from build123d import *

# Parameters (mm, degrees)
SKETCH1_R                 = 1.651
BOSS_EXTRUDE2_DEPTH       = 3.048
SKETCH2_R                 = 1.143
CUT_EXTRUDE1_DEPTH        = 4.048
SKETCH3_R                 = 12.1285
CUT_EXTRUDE2_DEPTH        = 4.048
SKETCH4_W                 = 28.562713242
SKETCH4_H                 = 11.677503754
BOSS_EXTRUDE3_DEPTH       = 3.048
SKETCH5_W                 = 216.7214489
SKETCH5_H                 = 130.569220634
CUT_EXTRUDE4_DEPTH        = 4.048
SKETCH6_W                 = 4.7625
SKETCH6_H                 = 27.432
CUT_EXTRUDE5_DEPTH        = 4.048
SKETCH10_W                = 11.43
SKETCH10_H                = 10.16
CUT_EXTRUDE9_DEPTH        = 4.048
FILLET1_R                 = 6
FILLET2_R                 = 6
SKETCH66_R                = 1.651
CUT_EXTRUDE65_DEPTH       = 97.79
SKETCH120_R               = 3.175
CUT_EXTRUDE119_DEPTH      = 103.378
CUT_EXTRUDE119_DEPTH_BACK = 48.768
CUT_EXTRUDE12_DEPTH       = 10
FILLET3_R                 = 2.54
BOSS_EXTRUDE4_DEPTH       = 3.048
SKETCH122_R               = 2.032
CUT_EXTRUDE120_DEPTH      = 27.305
SKETCH123_R               = 12.192
CUT_EXTRUDE121_DEPTH      = 19.05


with BuildPart() as part:
    # Sketch1 → Boss-Extrude2 (new body)
    with BuildSketch(Plane.XY):
        with BuildLine():
            Line((-64.964441474, 37.338), (-54.550441474, 37.338))
            Line((-54.550441474, 37.338), (-54.550441474, -37.338))
            Line((-54.550441474, -37.338), (-64.964441474, -37.338))
            ThreePointArc((-64.964441474, -37.338), (0, -74.93), (64.964441474, -37.338))
            Line((64.964441474, -37.338), (54.550441474, -37.338))
            Line((54.550441474, -37.338), (54.550441474, 37.338))
            Line((54.550441474, 37.338), (64.964441474, 37.338))
            ThreePointArc((64.964441474, 37.338), (0, 74.93), (-64.964441474, 37.338))
        make_face()
        with Locations((-46.482, 11.049)):
            Circle(SKETCH1_R, mode=Mode.SUBTRACT)
        with Locations((-21.083270032, 10.795)):
            Circle(SKETCH1_R, mode=Mode.SUBTRACT)
        with Locations((-21.083270032, -10.795)):
            Circle(SKETCH1_R, mode=Mode.SUBTRACT)
        with Locations((-46.482, -11.049)):
            Circle(SKETCH1_R, mode=Mode.SUBTRACT)
        with Locations((46.482, -11.049)):
            Circle(SKETCH1_R, mode=Mode.SUBTRACT)
        with Locations((21.083270032, -10.795)):
            Circle(SKETCH1_R, mode=Mode.SUBTRACT)
        with Locations((21.083270032, 10.795)):
            Circle(SKETCH1_R, mode=Mode.SUBTRACT)
        with Locations((46.482, 11.049)):
            Circle(SKETCH1_R, mode=Mode.SUBTRACT)
    extrude(amount=BOSS_EXTRUDE2_DEPTH)

    # Sketch2 → Cut-Extrude1 (cut, through all)
    with BuildSketch(Plane.XY.offset(3.048)):
        with Locations((-6.731, 62.23)):
            Circle(SKETCH2_R)
        with Locations((6.731, 62.23)):
            Circle(SKETCH2_R)
    extrude(amount=-CUT_EXTRUDE1_DEPTH, mode=Mode.SUBTRACT)

    # Sketch3 → Cut-Extrude2 (cut, through all)
    with BuildSketch(Plane(origin=(0, 0, 0), x_dir=(-1, 0, 0), z_dir=(0, 0, -1))):
        with Locations((-15.777608989, -58.882838371)):
            Circle(SKETCH3_R)
        with Locations((15.777608989, -58.882838371)):
            Circle(SKETCH3_R)
        with Locations((-43.105229381, -43.105229381)):
            Circle(SKETCH3_R)
        with Locations((19.05, 32.995567884)):
            Circle(SKETCH3_R)
        with Locations((-43.105229381, 43.105229381)):
            Circle(SKETCH3_R)
        with Locations((43.105229381, 43.105229381)):
            Circle(SKETCH3_R)
        with Locations((-19.05, 32.995567884)):
            Circle(SKETCH3_R)
        with Locations((43.105229381, -43.105229381)):
            Circle(SKETCH3_R)
    extrude(amount=-CUT_EXTRUDE2_DEPTH, mode=Mode.SUBTRACT)

    # Sketch4 → Boss-Extrude3 (add)
    with BuildSketch(Plane(origin=(0, 0, 0), x_dir=(-1, 0, 0), z_dir=(0, 0, -1))):
        with Locations((-1.488809975, 62.152540216)):
            Rectangle(SKETCH4_W, SKETCH4_H)
    extrude(amount=-BOSS_EXTRUDE3_DEPTH)

    # Sketch5 → Cut-Extrude4 (cut, through all)
    with BuildSketch(Plane(origin=(0, 0, 0), x_dir=(-1, 0, 0), z_dir=(0, 0, -1))):
        with Locations((23.316688373, 48.139610317)):
            Rectangle(SKETCH5_W, SKETCH5_H)
    extrude(amount=-CUT_EXTRUDE4_DEPTH, mode=Mode.SUBTRACT)

    # Sketch6 → Cut-Extrude5 (cut, through all)
    with BuildSketch(Plane(origin=(0, 0, 0), x_dir=(-1, 0, 0), z_dir=(0, 0, -1))):
        with Locations((0, -45.847)):
            Rectangle(SKETCH6_W, SKETCH6_H)
        Polygon((-2.38125, -34.131), (-2.38125, -32.131), (-6.38125, -32.131), (-6.38125, -17.145), (-9.38125, -17.145), (-9.38125, -34.131), align=None)
    extrude(amount=-CUT_EXTRUDE5_DEPTH, mode=Mode.SUBTRACT)

    # Sketch10 → Cut-Extrude9 (cut, through all)
    with BuildSketch(Plane(origin=(0, 0, 0), x_dir=(-1, 0, 0), z_dir=(0, 0, -1))):
        with Locations((-33.595441474, -22.225)):
            Rectangle(SKETCH10_W, SKETCH10_H)
        with Locations((33.595441474, -22.225)):
            Rectangle(SKETCH10_W, SKETCH10_H)
    extrude(amount=-CUT_EXTRUDE9_DEPTH, mode=Mode.SUBTRACT)

    # Fillet1
    fillet1_edges = [part.edges().sort_by_distance(p)[0] for p in [
        (6.38125, -32.131, 1.524),
    ]]
    fillet(fillet1_edges, radius=FILLET1_R)

    # Fillet2
    fillet2_edges = [part.edges().sort_by_distance(p)[0] for p in [
        (2.38125, -34.131, 1.524),
    ]]
    fillet(fillet2_edges, radius=FILLET2_R)

    # Sketch66 → Cut-Extrude65 (cut)
    with BuildSketch(Plane(origin=(30.092005081, 4.08352975, -16.1925), x_dir=(-1, 0, 0), z_dir=(0, 0, -1))):
        with Locations((4.154396091, -49.728759131)):
            Circle(SKETCH66_R)
        with Locations((56.02961407, -49.728759131)):
            Circle(SKETCH66_R)
    extrude(amount=-CUT_EXTRUDE65_DEPTH, mode=Mode.SUBTRACT)

    # Sketch120 → Cut-Extrude119 (cut, two sides)
    with BuildSketch(Plane(origin=(30.092005081, 4.08352975, 19.939), x_dir=(-1, 0, 0), z_dir=(0, 0, -1))) as cut_extrude119_sk:
        with Locations((77.082005081, -29.48352975)):
            Circle(SKETCH120_R)
        with Locations((30.092005081, -29.48352975)):
            Circle(SKETCH120_R)
        with Locations((-16.897994919, -29.48352975)):
            Circle(SKETCH120_R)
    extrude(amount=CUT_EXTRUDE119_DEPTH, mode=Mode.SUBTRACT)
    extrude(cut_extrude119_sk.sketch, amount=-CUT_EXTRUDE119_DEPTH_BACK, mode=Mode.SUBTRACT)

    # Sketch13 → Cut-Extrude12 (cut)
    with BuildSketch(Plane(origin=(0, 0, 0), x_dir=(-1, 0, 0), z_dir=(0, 0, -1))):
        with BuildLine():
            Line((-12.7, -20.24), (-8.888991966, -20.24))
            ThreePointArc((-8.888991966, -20.24), (-5.715, -23.495), (-2.541008034, -20.24))
            Line((-2.541008034, -20.24), (2.541008034, -20.24))
            ThreePointArc((2.541008034, -20.24), (5.715, -23.495), (8.888991966, -20.24))
            Line((8.888991966, -20.24), (12.7, -20.24))
            ThreePointArc((12.7, -20.24), (16.235533906, -11.704466094), (7.7, -15.24))
            Line((7.7, -15.24), (-1.0625, -15.24))
            ThreePointArc((-1.0625, -15.24), (-4.012347567, -10.679640913), (-9.38125, -11.500227489))
            ThreePointArc((-9.38125, -11.500227489), (-17.374337523, -13.465015853), (-12.7, -20.24))
        make_face()
    extrude(amount=-CUT_EXTRUDE12_DEPTH, mode=Mode.SUBTRACT)

    # Fillet3
    fillet3_edges = [part.edges().sort_by_distance(p)[0] for p in [
        (39.310441474, -17.145, 1.524),
        (27.880441474, -17.145, 1.524),
        (-27.880441474, -17.145, 1.524),
        (-39.310441474, -17.145, 1.524),
        (6.38125, -23.424309253, 1.524),
        (9.38125, -20.24, 1.524),
        (17.322875188, -17.145, 1.524),
        (-17.322875188, -17.145, 1.524),
        (-8.888991966, -20.24, 1.524),
        (-2.541008034, -20.24, 1.524),
        (2.541008034, -20.24, 1.524),
    ]]
    fillet(fillet3_edges, radius=FILLET3_R)

    # Sketch121 → Boss-Extrude4 (add)
    with BuildSketch(Plane.XY.offset(3.048)):
        with BuildLine():
            Line((2.891074229, -60.515426156), (4.322679041, -42.124810499))
            Line((4.322679041, -42.124810499), (14.013542381, -30.56184856))
            Line((14.013542381, -30.56184856), (14.76082601, -20.962128091))
            Line((14.76082601, -20.962128091), (16.738759609, -18.187612732))
            ThreePointArc((16.738759609, -18.187612732), (14.965164049, -19.697469218), (12.7, -20.24))
            Line((12.7, -20.24), (10.873451803, -20.24))
            ThreePointArc((10.873451803, -20.24), (9.5179937, -20.631900064), (8.580806557, -21.686666667))
            ThreePointArc((8.580806557, -21.686666667), (5.715, -23.495), (2.849193443, -21.686666667))
            Line((2.849193443, -21.686666667), (4.942864205, -26.845073773))
            Line((4.942864205, -26.845073773), (2.891074229, -29.631036754))
            Line((2.891074229, -29.631036754), (-4.156826382, -31.552959583))
            Line((-4.156826382, -31.552959583), (-2.945468464, -62.167277862))
            Line((-2.945468464, -62.167277862), (2.891074229, -60.515426156))
        make_face()
    extrude(amount=-BOSS_EXTRUDE4_DEPTH)

    # Sketch122 → Cut-Extrude120 (cut)
    with BuildSketch(Plane.XY.offset(3.048)):
        with Locations((0, -50.165)):
            Circle(SKETCH122_R)
    extrude(amount=-CUT_EXTRUDE120_DEPTH, mode=Mode.SUBTRACT)

    # Sketch123 → Cut-Extrude121 (cut)
    with BuildSketch(Plane(origin=(0, 0, 0), x_dir=(-1, 0, 0), z_dir=(0, 0, -1))):
        with Locations((-15.777608989, -33.482838371)):
            Circle(SKETCH123_R)
        with Locations((15.777608989, -33.482838371)):
            Circle(SKETCH123_R)
    extrude(amount=-CUT_EXTRUDE121_DEPTH, mode=Mode.SUBTRACT)


solid = part.part
Here's how the part is built. I have some questions about the finished solid (model axes, mm). A direction names the side the tool comes from. Round coordinates to 2 decimals unless told otherwise and drop trailing zeros. Write each loop counter-clockwise with the first axis right and the second up, starting at its lowest first coordinate (ties: lowest second). Pieces come first, ordered by that corner, then holes.
1. Suppose I cut it at A-A (x = 45). List the corners of the cut face in (y, z) for me (3 decimals).
2. Suppose I cut it at B-B (y = -39). List the corners of the cut face in (x, z) for me, and give its area (3 significant figures).
3. Suppose I cut it at D-D (y = -68). List the corners of the cut face in (x, z) for me, and give its area (3 significant figures).
4. For faces 5 (the cylindrical face through (-14.94, -19.71, 1.5)), 6 (the flat face through (60, -37.338, 2)), 7 (the cylindrical face through (-24.63, -46.65, 1.5)), which set-ups out of +Z, -Z, +X, -X, +Y, -Y let a thin tool reach every point of the face, with its end or its side?
5. If we mould it in two halves opening along X, with no side actions, what happens to faces 1 (the flat face through (-48, -17.145, 2)), 2 (the cylindrical face through (-1.1, -74.92, 1.5)), 3 (the flat face through (-54.55, -27, 2)), 4 (the cylindrical face through (-50.02, -24.45, 1.55))? For each: released by +X, released by -X, zero draft, split by the parting line, or undercut.
6. I need wall thicknesses on L1, parallel to Y at x = -17.5, z = 2.3; L2, parallel to Y at x = -11, z = 0.3; L3, parallel to X at y = -67, z = 0.7. Which ranges of each line are inside material? Lowest first, please.
7. Will these pins go through, and if not, where does the flat tip stop? pin 1 Ø1.5 at (y, z) = (-25, 2) entering from -X; pin 2 Ø0.9 at (y, z) = (-25, 1) entering from +X.
8. Suppose I cut it at C-C (y = -25.4). State how many separate pieces and enclosed holes the cut face has, and give its area (3 significant figures).
Answer sheet:
1. outline: (-59.912, 0) - (-55.085, 0) - (-55.085, 3.048) - (-59.912, 3.048) - close; (-31.126, 0) - (-27.874, 0) - (-27.874, 3.048) - (-31.126, 3.048) - close; (-22.926, 0) - (-17.145, 0) - (-17.145, 3.048) - (-22.926, 3.048) - close
2. outline: (-63.98, 0) - (-54.52, 0) - (-54.52, 3.05) - (-63.98, 3.05) - close; (-31.69, 0) - (-26.65, 0) - (-26.65, 3.05) - (-31.69, 3.05) - close; (-4.91, 0) - (4.91, 0) - (4.91, 3.05) - (-4.91, 3.05) - close; (26.65, 0) - (31.69, 0) - (31.69, 3.05) - (26.65, 3.05) - close; (54.52, 0) - (63.98, 0) - (63.98, 3.05) - (54.52, 3.05) - close
2. area: 118 mm2
3. outline: (-31.47, 0) - (-23.78, 0) - (-23.78, 3.05) - (-31.47, 3.05) - close; (-7.78, 0) - (7.78, 0) - (7.78, 3.05) - (-7.78, 3.05) - close; (23.78, 0) - (31.47, 0) - (31.47, 3.05) - (23.78, 3.05) - close
3. area: 94.3 mm2
4. face 5: +Z, -Z, +Y
4. face 6: +Z, -Z, +X, +Y
4. face 7: +Z, -Z
5. face 1: zero draft
5. face 2: split by the parting line
5. face 3: released by -X
5. face 4: undercut
6. L1: y = -72.86 to -70.89, -46.88 to -45.55, -21.41 to -17.5
6. L2: y = -74.12 to -70.03, -47.73 to -44.7, -22.27 to -20.24
6. L3: x = -33.55 to -24.79, -6.77 to 6.77, 24.79 to 33.55
7. pin 1: stops at x = -54.55
7. pin 2: stops at x = 54.55
8. separate pieces: 8
8. enclosed holes: 0
8. area: 93.5 mm2
